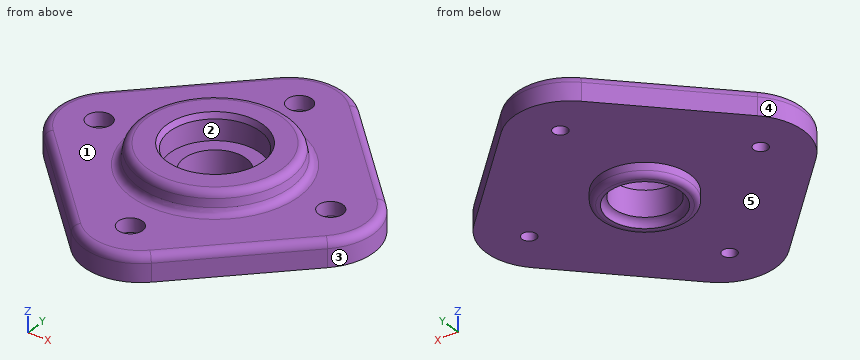
```python
from build123d import *

# Parameters (mm, degrees)
BOSS_EXTRUDE1_DEPTH     = 10
SKETCH2_R               = 30
BOSS_EXTRUDE2_DEPTH     = 8
BOSS_EXTRUDE2_TAPER     = 10
SKETCH4_R               = 17.5
BOSS_EXTRUDE3_DEPTH     = 5
CUT_EXTRUDE1_DEPTH      = 91.097848019
CUT_EXTRUDE1_DEPTH_BACK = 91.097848019
SKETCH3_R               = 12
SKETCH3_3_R             = 17.5
SKETCH3_3_R_2           = 12
CUT_EXTRUDE2_DEPTH      = 10
SKETCH5_R               = 14
CUT_EXTRUDE3_DEPTH      = 3
CUT_EXTRUDE4_DEPTH      = 89.394695642
CUT_EXTRUDE4_DEPTH_BACK = 89.394695642
SKETCH6_R               = 2.75
SKETCH6_3_R             = 4.75
SKETCH6_3_R_2           = 2.75
CUT_EXTRUDE5_DEPTH      = 5.4
FILLET1_R               = 3
FILLET2_R               = 3
FILLET3_R               = 3
FILLET4_R               = 2


with BuildPart() as part:
    # Sketch1 → Boss-Extrude1 (new body)
    with BuildSketch(Plane.XY):
        with BuildLine():
            Line((-15.556349186, 55.154328933), (-55.154328933, 15.556349186))
            ThreePointArc((-55.154328933, 15.556349186), (-61.597979746, 0), (-55.154328933, -15.556349186))
            Line((-55.154328933, -15.556349186), (-15.556349186, -55.154328933))
            ThreePointArc((-15.556349186, -55.154328933), (0, -61.597979746), (15.556349186, -55.154328933))
            Line((15.556349186, -55.154328933), (55.154328933, -15.556349186))
            ThreePointArc((55.154328933, -15.556349186), (61.597979746, 0), (55.154328933, 15.556349186))
            Line((55.154328933, 15.556349186), (15.556349186, 55.154328933))
            ThreePointArc((15.556349186, 55.154328933), (0, 61.597979746), (-15.556349186, 55.154328933))
        make_face()
    extrude(amount=BOSS_EXTRUDE1_DEPTH)

    # Sketch2 → Boss-Extrude2 (add)
    with BuildSketch(Plane.XY.offset(10)):
        Circle(SKETCH2_R)
    extrude(amount=BOSS_EXTRUDE2_DEPTH, taper=BOSS_EXTRUDE2_TAPER)

    # Sketch4 → Boss-Extrude3 (add)
    with BuildSketch(Plane(origin=(0, 0, 0), x_dir=(-1, 0, 0), z_dir=(0, 0, -1))):
        Circle(SKETCH4_R)
    extrude(amount=BOSS_EXTRUDE3_DEPTH)

    # Sketch3 → Cut-Extrude1 (cut, two sides: drawn at the far end of the back side and taken through both)
    with BuildSketch(Plane.XY.offset(18).offset(-CUT_EXTRUDE1_DEPTH_BACK)):
        Circle(SKETCH3_R)
    extrude(amount=CUT_EXTRUDE1_DEPTH + CUT_EXTRUDE1_DEPTH_BACK, mode=Mode.SUBTRACT)

    # Sketch3<3> → Cut-Extrude2 (cut)
    with BuildSketch(Plane.XY.offset(18)):
        with Locations(Location((0, 0, 0), (0, 0, 180))):
            Circle(SKETCH3_3_R)
        Circle(SKETCH3_3_R_2, mode=Mode.SUBTRACT)
    extrude(amount=-CUT_EXTRUDE2_DEPTH, mode=Mode.SUBTRACT)

    # Sketch5 → Cut-Extrude3 (cut)
    with BuildSketch(Plane(origin=(0, 0, -5), x_dir=(-1, 0, 0), z_dir=(0, 0, -1))):
        Circle(SKETCH5_R)
    extrude(amount=-CUT_EXTRUDE3_DEPTH, mode=Mode.SUBTRACT)

    # Sketch6 → Cut-Extrude4 (cut, two sides: drawn at the far end of the back side and taken through both)
    with BuildSketch(Plane.XY.offset(10).offset(-CUT_EXTRUDE4_DEPTH_BACK)):
        with Locations((0, 45)):
            Circle(SKETCH6_R)
        with Locations((45, 0)):
            Circle(SKETCH6_R)
        with Locations((0, -45)):
            Circle(SKETCH6_R)
        with Locations((-45, 0)):
            Circle(SKETCH6_R)
    extrude(amount=CUT_EXTRUDE4_DEPTH + CUT_EXTRUDE4_DEPTH_BACK, mode=Mode.SUBTRACT)

    # Sketch6<3> → Cut-Extrude5 (cut)
    # profile 1 of 4: a face of its own
    with BuildSketch(Plane.XY.offset(10)):
        with Locations((-45, 0)):
            Circle(SKETCH6_3_R)
        with Locations((-45, 0)):
            Circle(SKETCH6_3_R_2, mode=Mode.SUBTRACT)
    # profile 2 of 4: a face of its own
    with BuildSketch(Plane.XY.offset(10)):
        with Locations((0, -45)):
            Circle(SKETCH6_3_R)
        with Locations((0, -45)):
            Circle(SKETCH6_3_R_2, mode=Mode.SUBTRACT)
    # profile 3 of 4: a face of its own
    with BuildSketch(Plane.XY.offset(10)):
        with Locations((45, 0)):
            Circle(SKETCH6_3_R)
        with Locations((45, 0)):
            Circle(SKETCH6_3_R_2, mode=Mode.SUBTRACT)
    # profile 4 of 4: a face of its own
    with BuildSketch(Plane.XY.offset(10)):
        with Locations((0, 45)):
            Circle(SKETCH6_3_R)
        with Locations((0, 45)):
            Circle(SKETCH6_3_R_2, mode=Mode.SUBTRACT)
    extrude(amount=-CUT_EXTRUDE5_DEPTH, mode=Mode.SUBTRACT)

    # Sketch7 → Cut-Revolve1 (revolve, cut)
    with BuildSketch(Plane(origin=(0, 0, 0), x_dir=(0, 0, -1), z_dir=(1, 0, 0)), mode=Mode.PRIVATE) as cut_revolve1_sk:
        Polygon((-18, 17.5), (-16, 17.5), (-18, 18.654700538), align=None)
    revolve(cut_revolve1_sk.sketch.rotate(Axis((0, 0, 32.778670792), (0, 0, -1)), 90), axis=Axis((0, 0, 32.778670792), (0, 0, -1)), mode=Mode.SUBTRACT)

    # Fillet1
    fillet1_edges = [part.edges().sort_by_distance(p)[0] for p in [
        (-30, 0, 10),
        (-28.589384154, 0, 18),
    ]]
    fillet(fillet1_edges, radius=FILLET1_R)

    # Fillet2
    fillet2_edges = [part.edges().sort_by_distance(p)[0] for p in [
        (61.597979746, 0, 10),
        (35.355339059, 35.355339059, 10),
        (0, 61.597979746, 10),
        (-35.355339059, 35.355339059, 10),
        (-61.597979746, 0, 10),
        (-35.355339059, -35.355339059, 10),
        (0, -61.597979746, 10),
        (35.355339059, -35.355339059, 10),
    ]]
    fillet(fillet2_edges, radius=FILLET2_R)

    # Fillet3
    # the kernel refuses this fillet: 3 mm, written as the material it adds along each edge
    with BuildSketch(Plane(origin=(0, 0, -2), x_dir=(-1, 0, 0), z_dir=(0, -1, 0))) as fillet3_piece_1:
        with BuildLine():
            CenterArc((11, 2.828427125), FILLET3_R, 289.471220634, 70.528779366)
            Line((12, 0), (12.02, -0.056568542))
            ThreePointArc((12.02, -0.056568542), (13, -0.06), (14, -0.06))
            Line((14, -0.06), (14.06, 0))
            Line((14.06, 0), (14.06, 2.828427125))
            Line((14.06, 2.828427125), (14, 2.828427125))
        make_face()
    revolve(axis=Axis((0, 0, -2), (0, 0, -1)))

    # Fillet4
    fillet4_edges = [part.edges().sort_by_distance(p)[0] for p in [
        (17.5, 0, -5),
    ]]
    fillet(fillet4_edges, radius=FILLET4_R)


solid = part.part
```
CAD build for the part. Positions are in the model's coordinates, mm. Face numbers are marked on the shaded views. A direction names the side the tool comes from. Coordinates: 2 decimals unless noted, no trailing zeros. Write each loop counter-clockwise with the first axis right and the second up, starting at its lowest first coordinate (ties: lowest second). Pieces come first, ordered by that corner, then holes. Notation, with made-up numbers: (11.25, 13) -> (70.25, 13) arc R25 ccw to (70.25, 41) -> close; hole circle Ø6 at (-2, 11.5). An arc over 180 degrees is marked (long way). Use CSV: the item, a comma, the result in double quotes. Start each with the question number.
Item 1: Drop flat-ended pins along their axis: P1, Ø9, axis at x = 0, y = 45, coming from the +Z side; P2, Ø2, axis at y = -9.5, z = 3.5, coming from the -X side; P3, Ø11, axis at x = 45, y = 0, coming from the +Z side; P4, Ø4.5, axis at x = 45, y = 0, coming from the -Z side. Give the stop position or say it passes through.
Item 2: Band-saw the part on A-A, the plane z = 2. Write the cut outline in (x, y).
Item 3: Wall check: probe 1 along X at (y, z) = (0, 0.5); probe 2 along Z at (x, y) = (-11, 21). Give the ranges that are in metal, low to high.
Item 4: Two-plate mould, pull along X, no slides. Class the marked faces 1, 2 and 3: +X half, -X half, draft (parallel to the pull), parting line (faces both ways), or undercut.
Item 5: Tool access for the marked faces 4 and 5: list every direction of +Z, -Z, +X, -X, +Y, -Y with a clear straight run to the whole face (end or side of a thin tool).
Item 6: Band-saw the part on B-B, the plane y = 0. Give the number of separate pieces and of enclosed holes in the cut face, plus the area to 3 significant figures.
Response values:
1,P1,"stops at z = 4.6"
1,P2,"stops at x = -59.89"
1,P3,"stops at z = 10"
1,P4,"passes through"
2,outline,"(-55.15, -15.56) -> (-15.56, -55.15) arc R22 ccw to (15.56, -55.15) -> (55.15, -15.56) arc R22 ccw to (55.15, 15.56) -> (15.56, 55.15) arc R22 ccw to (-15.56, 55.15) -> (-55.15, 15.56) arc R22 ccw to start; hole circle Ø5.5 at (-45, 0); hole circle Ø24 at (0, 0); hole circle Ø5.5 at (0, -45); hole circle Ø5.5 at (0, 45); hole circle Ø5.5 at (45, 0)"
3,probe 1,"x = -61.6 to -47.75, -42.25 to -12, 12 to 42.25, 47.75 to 61.6"
3,probe 2,"z = 0 to 18"
4,face 1,"draft"
4,face 2,"undercut"
4,face 3,"+X half"
5,face 4,"+Z, -Z, -X"
5,face 5,"-Z"
6,separate pieces,"4"
6,enclosed holes,"0"
6,area,"1,040 mm2"
